Check sheet for the modelled part. Datum: model origin and axes. Units: mm. Give positions to 0.01 mm unless a question says otherwise; leave off trailing zeros. Order: outer loops, then holes, each group sorted by start corner. A loop starts at its lowest first (then second) coordinate and runs counter-clockwise, first axis right, second up.
```python
from build123d import *

# Parameters (mm, degrees)
DODANIE_WYCI_GNI_CIE1_DEPTH = 10
SZKIC2_R                    = 1.5
WYTNIJ_WYCI_GNI_CIE1_DEPTH  = 10
SZKIC5_R                    = 5.075
WYTNIJ_WYCI_GNI_CIE2_DEPTH  = 10
WYTNIJ_WYCI_GNI_CIE3_DEPTH  = 10
DODANIE_WYCI_GNI_CIE2_DEPTH = 10


with BuildPart() as part:
    # Szkic1 → Dodanie-wyciągnięcie1 (new body)
    with BuildSketch(Plane.XY):
        with BuildLine():
            Line((656.238844698, -438.745595983), (352.638844698, -438.745595983))
            ThreePointArc((352.638844698, -438.745595983), (348.113361298, -436.871079382), (346.238844698, -432.345595983))
            Line((346.238844698, -432.345595983), (346.238844698, -405.145595983))
            ThreePointArc((346.238844698, -405.145595983), (348.113361298, -400.620112583), (352.638844698, -398.745595983))
            Line((352.638844698, -398.745595983), (394.238844698, -398.745595983))
            Line((394.238844698, -398.745595983), (397.838844698, -398.745595983))
            ThreePointArc((397.838844698, -398.745595983), (402.364328097, -400.620112583), (404.238844698, -405.145595983))
            Line((404.238844698, -405.145595983), (404.238844698, -411.345595983))
            ThreePointArc((404.238844698, -411.345595983), (402.364328097, -415.871079382), (397.838844698, -417.745595983))
            Line((397.838844698, -417.745595983), (394.238844698, -417.745595983))
            Line((394.238844698, -417.745595983), (394.238844698, -424.745595983))
            Line((394.238844698, -424.745595983), (656.238844698, -424.745595983))
            Line((656.238844698, -424.745595983), (656.238844698, -438.745595983))
        make_face()
    extrude(amount=DODANIE_WYCI_GNI_CIE1_DEPTH)

    # Szkic2 → Wytnij-wyciągnięcie1 (cut)
    with BuildSketch(Plane.XY.offset(10)):
        with Locations((644.238844698, -430.4368906)):
            Circle(SZKIC2_R)
        with Locations((592.238844698, -430.4368906)):
            Circle(SZKIC2_R)
        with Locations((540.238844698, -430.4368906)):
            Circle(SZKIC2_R)
        with Locations((488.238844698, -430.4368906)):
            Circle(SZKIC2_R)
        with Locations((436.238844698, -430.4368906)):
            Circle(SZKIC2_R)
        with Locations((384.238844698, -430.4368906)):
            Circle(SZKIC2_R)
        with Locations((356.238844698, -430.4368906)):
            Circle(SZKIC2_R)
        with Locations((399.238844698, -408.245595983)):
            Circle(SZKIC2_R)
    extrude(amount=-WYTNIJ_WYCI_GNI_CIE1_DEPTH, mode=Mode.SUBTRACT)

    # Szkic5 → Wytnij-wyciągnięcie2 (cut)
    with BuildSketch(Plane(origin=(0, 0, 0), x_dir=(-1, 0, 0), z_dir=(0, 0, -1))):
        with Locations((-364.238844698, -407.745595983)):
            Circle(SZKIC5_R)
    extrude(amount=-WYTNIJ_WYCI_GNI_CIE2_DEPTH, mode=Mode.SUBTRACT)

    # Szkic6 → Wytnij-wyciągnięcie3 (cut)
    with BuildSketch(Plane(origin=(0, 0, 0), x_dir=(-1, 0, 0), z_dir=(0, 0, -1))):
        with BuildLine():
            Line((-656.238844698, -430.745595983), (-656.238844698, -424.745595983))
            Line((-656.238844698, -424.745595983), (-650.238844698, -424.745595983))
            ThreePointArc((-650.238844698, -424.745595983), (-654.481485385, -426.502955296), (-656.238844698, -430.745595983))
        make_face()
    extrude(amount=-WYTNIJ_WYCI_GNI_CIE3_DEPTH, mode=Mode.SUBTRACT)

    # Szkic7 → Dodanie-wyciągnięcie2 (add)
    with BuildSketch(Plane.XY.offset(10)):
        with BuildLine():
            Line((624.50679389, -424.745595983), (627.970895505, -424.745595983))
            ThreePointArc((627.970895505, -424.745595983), (627.470895505, -424.611621386), (627.104870102, -424.245595983))
            ThreePointArc((627.104870102, -424.245595983), (626.238844698, -423.745595983), (625.372819294, -424.245595983))
            ThreePointArc((625.372819294, -424.245595983), (625.00679389, -424.611621386), (624.50679389, -424.745595983))
        make_face()
    extrude(amount=-DODANIE_WYCI_GNI_CIE2_DEPTH)


solid = part.part
```
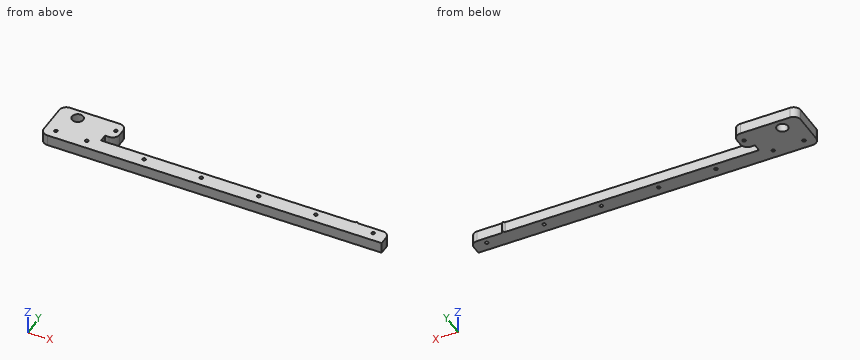
(1) Sectioned sample at B-B (x = 551). Enter the section's corners in (y, z), plus the area to 3 significant figures.
(2) Thickness scan on L1, parallel to Y at x = 396, z = 6.5; L2, parallel to X at y = -408, z = 8.75; L3, parallel to Y at x = 589.5, z = 1.25. Record the ranges inside material, lowest first.
(3) Sectioned sample at A-A (z = 7). Count the separate pieces of the cut face and the enclosed holes in it, plus the area to 3 significant figures.
(4) Go/stop test with flat-tipped pins: P1, Ø1, axis at x = 575.5, z = 2, coming from the +Y side; P2, Ø5.5, axis at y = -420, z = 6.5, coming from the +X side. Record where each tip stops, or that it passes through.
Values follow:
1. outline: (-438.75, 0) - (-424.75, 0) - (-424.75, 10) - (-438.75, 10) - close
1. area: 140 mm2
2. L1: y = -438.75 to -424.75, -417.75 to -398.75
2. L2: x = 346.24 to 359.17, 369.31 to 397.76, 400.72 to 404.24
2. L3: y = -438.75 to -424.75
3. separate pieces: 1
3. enclosed holes: 9
3. area: 5,600 mm2
4. P1: stops at y = -424.75
4. P2: stops at x = 400.31
